```python
from build123d import *

# Parameters (mm, degrees)
SKETCH1_R           = 13.462
BOSS_EXTRUDE1_DEPTH = 31.75
SKETCH2_R           = 11.43
BOSS_EXTRUDE2_DEPTH = 31.75
SKETCH3_R           = 3.175
CUT_EXTRUDE1_DEPTH  = 25.4


# Read off the part's stored shape, not the designer's step: 7/16-14 Machine Threads Stud1
with BuildPart() as part:
    # Sketch1 → Boss-Extrude1 (new body)
    with BuildSketch(Plane.XY):
        Circle(SKETCH1_R)
    extrude(amount=BOSS_EXTRUDE1_DEPTH)

    # Sketch2 → Boss-Extrude2 (add)
    with BuildSketch(Plane.XY.offset(31.75)):
        Circle(SKETCH2_R)
    extrude(amount=BOSS_EXTRUDE2_DEPTH)

    # Sketch3 → Cut-Extrude1 (cut)
    with BuildSketch(Plane.XY.offset(63.5)):
        Circle(SKETCH3_R)
    extrude(amount=-CUT_EXTRUDE1_DEPTH, mode=Mode.SUBTRACT)

    # 7/16-14 Machine Threads Stud1 outline → 7/16-14 Machine Threads Stud1 (revolve)
    with BuildSketch(Plane.XZ):
        Polygon((0, 0), (0, -25.4), (4.47675, -25.4), (5.55625, -24.3205), (5.55625, 0), align=None)
    revolve(axis=Axis((0, 0, 0), (0, 0, 1)))


solid = part.part
```
Build history of the part. All positions in model axes, mm. A direction names the side the tool comes from. Coordinates: 2 decimals unless noted, no trailing zeros. Order: outer loops, then holes, each group sorted by start corner. A loop starts at its lowest first (then second) coordinate and runs counter-clockwise, first axis right, second up. Notation, with made-up numbers: (-16.5, -16.5) -> (41.5, -16.5) arc R16 ccw to (41.5, -9.5) -> close; hole circle Ø3 at (72, 69.25). An arc over 180 degrees is marked (long way). Answer in a Markdown table with one row per item. Add a question column.
Q1. Drop flat-ended pins along their axis: pin 1 (8 mm diameter, centred on y = -5.5, z = 23.5, fed in from -X); pin 2 (12 mm diameter, centred on y = -9.5, z = 54, fed in from +X); pin 3 (1.9 mm diameter, centred on x = 0, y = 1, fed in from +Z). Give the stop position or say it passes through.
Q2. Which spindle directions (+Z, -Z, +X, -X, +Y, -Y) get a long thin tool onto all of the face, cutting with end or side? Do faces 5 (the face through (-6, -10, 31.75)), 6 (the face through (-10.683, -8.191, 15.653)), 7 (the face through (6, 0, 0)). Say none if no direction does.
Q3. Wall check: line 1 along Y through (x, z) = (0, 50.75) (3 decimals); line 2 along Z through (x, y) = (-10.25, -3.75); line 3 along Z through (x, y) = (1.5, -1.25). Give the ranges that are in metal, low to high. Write a range as [from, to].
Q4. Band-saw the part on D-D, the plane z = -7. List the corners of the cut face in (x, y), then the cut area to 3 significant figures.
Q5. Mould opens along X. For faces 1 (the face through (0, 0, 38.1)), 2 (the face through (10.902, 3.433, 47.403)), 3 (the face through (-0.69, -3.1, 50.98)), 4 (the face through (2.4, -2.4, 63.5)) say: +X half, -X half, draft (parallel to the pull), parting line (faces both ways), or undercut.
Q6. Band-saw the part on C-C, the plane z = 53. List the corners of the cut face in (x, y) (3 decimals).
Answers follow:
| question | item | result |
|---|---|---|
| 1 | pin 1 | x = -13.38 |
| 1 | pin 2 | x = 10.88 |
| 1 | pin 3 | z = 38.1 |
| 2 | face 5 | +Z |
| 2 | face 6 | +Z, -Z |
| 2 | face 7 | -Z |
| 3 | line 1 | [-11.43, -3.175], [3.175, 11.43] |
| 3 | line 2 | [0, 63.5] |
| 3 | line 3 | [-25.4, 38.1] |
| 4 | outline | circle Ø11.11 at (0, 0) |
| 4 | area | 97.0 mm^2 |
| 5 | face 1 | undercut |
| 5 | face 2 | parting line |
| 5 | face 3 | undercut |
| 5 | face 4 | draft |
| 6 | outline | circle Ø22.86 at (0, 0); hole circle Ø6.35 at (0, 0) |
